The figure shows three views and two pictorial views of one solid part (mm, origin at its lowest corner). Answer the questions. Give positions to 0.01 mm unless a question says otherwise; leave off trailing zeros. Write each loop counter-clockwise with the first axis right and the second up, starting at its lowest first coordinate (ties: lowest second). Pieces come first, ordered by that corner, then holes. Notation, with made-up numbers: M 50.25,76.25 L 73.25,76.25 A26 cw 73.25,112.25 Z; hole C -34,68.5 d2. An arc over 180 degrees is marked long. Return JSON: item names as keys, results as strings.
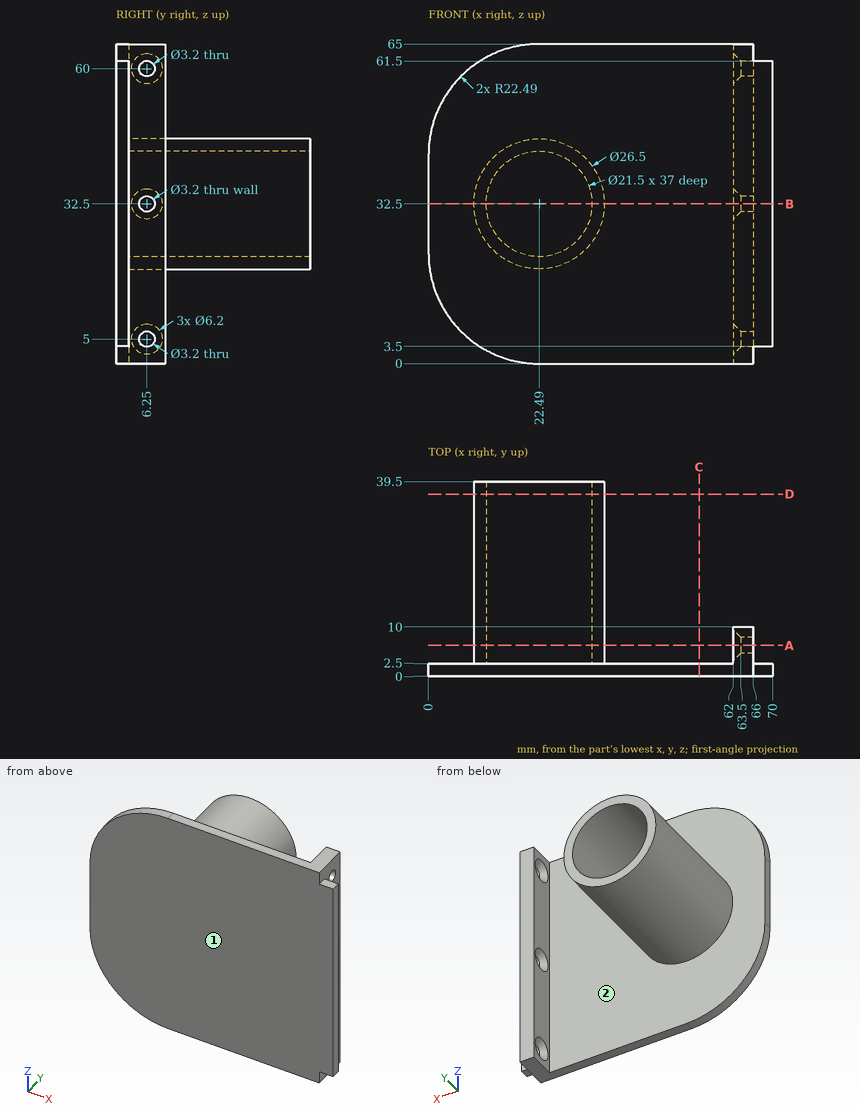
Item 1: A cutting plane is placed at C-C, the plane x = 55. Write down the section's boundary in (y, z), plus the area to 4 significant figures.
Geometry results:
{"outline": "M 0,0 L 2.5,0 L 2.5,65 L 0,65 Z", "area": "162.5 mm2"}
Item 2: Determine the mould class of the marked faces 1 and 2 for opening direction X: +X half, -X half, draft (parallel to the pull), parting line (faces both ways), or undercut.
Geometry results:
{"face 1": "draft", "face 2": "undercut"}
Item 3: Find the intervals of material crossed by line 1 (Z direction, x = 65, y = 6); line 2 (Z direction, x = 23, y = 7.5); line 3 (X direction, y = 32.5, z = 33), in increasing order.
Geometry results:
{"line 1": "z = 0 to 3.42, 6.58 to 30.92, 34.08 to 58.42, 61.58 to 65", "line 2": "z = 19.26 to 21.76, 43.24 to 45.74", "line 3": "x = 9.25 to 11.75, 33.23 to 35.73"}
Item 4: A cutting plane is placed at A-A, the plane y = 6.25. Write down the section's boundary in (x, z), plus the area to 3 significant figures.
Geometry results:
{"outline": "C 22.49,32.5 d26.5; M 62,0 L 66,0 L 66,3.4 L 63.5,3.4 L 62,1.9 Z; M 62,8.1 L 63.5,6.6 L 66,6.6 L 66,30.9 L 63.5,30.9 L 62,29.4 Z; M 62,35.6 L 63.5,34.1 L 66,34.1 L 66,58.4 L 63.5,58.4 L 62,56.9 Z; M 62,63.1 L 63.5,61.6 L 66,61.6 L 66,65 L 62,65 Z; hole C 22.49,32.5 d21.5", "area": "403 mm2"}
Item 5: A cutting plane is placed at D-D, the plane y = 37. Write down the section's boundary in (x, z).
Geometry results:
{"outline": "C 22.49,32.5 d26.5; hole C 22.49,32.5 d21.5"}
Item 6: Given pin 1 Ø2.5 at (y, z) = (6.25, 32.5) entering from -X; pin 2 Ø4 at (x, z) = (50, 12) entering from -Y; pin 3 Ø17 at (x, z) = (22.49, 32.5) entering from +Y; pin 4 Ø3 at (y, z) = (11.5, 23) entering from -X, each flat-ended and moving along its own axis, determine where each tip first touches the part or whether it passes through.
Geometry results:
{"pin 1": "stops at x = 9.24", "pin 2": "stops at y = 0", "pin 3": "stops at y = 2.5", "pin 4": "stops at x = 11.93"}
Item 7: A cutting plane is placed at B-B, the plane z = 32.5. Write down the section's boundary in (x, y).
Geometry results:
{"outline": "M 0,0 L 70,0 L 70,2.5 L 66,2.5 L 66,4.65 L 63.5,4.65 L 62,3.15 L 62,2.5 L 35.74,2.5 L 35.74,39.5 L 33.24,39.5 L 33.24,2.5 L 11.74,2.5 L 11.74,39.5 L 9.24,39.5 L 9.24,2.5 L 0,2.5 Z; M 62,9.35 L 63.5,7.85 L 66,7.85 L 66,10 L 62,10 Z"}
